```python
from build123d import *

# Parameters (mm, degrees)
EXTRUDE_DEPTH    = 5
EXTRUDE001_DEPTH = 25
EXTRUDE002_DEPTH = 22


with BuildPart() as extrude_body:
    # Sketch → Extrude (new body)
    with BuildSketch(Plane.XY):
        Polygon((115, 0), (57.5, 99.592921), (-57.5, 99.592921), (-115, 0), (-57.5, -99.592921), (57.5, -99.592921), align=None)
    extrude(amount=EXTRUDE_DEPTH)


with BuildPart() as extrude001:
    # Sketch001 (on Sketch) → Extrude001 (new body)
    with BuildSketch(Plane.XY):
        Polygon((115, 0), (57.5, 99.592921), (-57.5, 99.592921), (-115, 0), (-57.5, -99.592921), (57.5, -99.592921), align=None)
        Polygon((112.5, 0), (56.25, 97.427858), (-56.25, 97.427858), (-112.5, 0), (-56.25, -97.427858), (56.25, -97.427858), align=None, mode=Mode.SUBTRACT)
    extrude(amount=EXTRUDE001_DEPTH)


with BuildPart() as fusion:
    # Sketch002 (on Sketch) → Extrude002 (new body)
    with BuildSketch(Plane.XY):
        Polygon((112.5, 0), (56.25, 97.427858), (-56.25, 97.427858), (-112.5, 0), (-56.25, -97.427858), (56.25, -97.427858), align=None)
        Polygon((111, 0), (55.5, 96.12882), (-55.5, 96.12882), (-111, 0), (-55.5, -96.12882), (55.5, -96.12882), align=None, mode=Mode.SUBTRACT)
    extrude(amount=EXTRUDE002_DEPTH)

    # Fusion: union Extrude body, Extrude001
    add(extrude_body.part)
    add(extrude001.part)


solid = fusion.part
```
Source: CAD feature listing. Evaluate the final solid. Frame: model axes, mm. A direction names the side the tool comes from. Coordinates: 2 decimals unless noted, no trailing zeros. Loops run counter-clockwise (first coordinate to the right, second up) from the corner with the lowest first, then second, coordinate; pieces in that order, holes last. Notation, with made-up numbers: (56, 19.25) -> (79, 19.25) arc R18 cw to (79, 51.25) -> close; hole circle Ø10 at (4, 13.25). An arc over 180 degrees is marked (long way). One line per item, written item: value. Start each with the question number.
Q1. Section query B-B, the plane x = 18. Return the cut outline in (y, z), and give its area (3 significant figures).
Q2. Line query: line 1 along Y through (x, z) = (-45, 5.25); line 2 along Y through (x, z) = (56, 22.5); line 3 along Z through (x, y) = (18, 14). Output: solid intervals per line, ascending.
Q3. Mould query, pull axis Y, two halves, no side actions, for faces 1 (the face through (-83.64, -47.39, 13.38)), 2 (the face through (86.65, 49.1, 12.32)), 3 (the face through (-2, 1, 0)). Classes: pulls with the +Y half, pulls with the -Y half, needs draft (parallel to the pull), parting line crosses it, or undercut.
Q4. Contact query for flat-ended pins moving along their axis: P1, Ø8, axis at x = 67, z = 17.5, coming from the +Y side; P2, Ø8, axis at y = -11.5, z = 2.5, coming from the +X side; P3, Ø5, axis at x = 89, z = 22.5, coming from the +Y side. Output: stop coordinate, or through.
Q5. Section query C-C, the plane y = -69. Return the cut outline in (x, z).
Q6. Set-up query: faces 4 (the face through (84.77, 48.03, 23.48)), 5 (the face through (-85.85, 50.49, 12.32)). Return all of +Z, -Z, +X, -X, +Y, -Y with unobstructed straight access to the full face (end or side cutting, diameter ignored); none if empty.
Q7. Section query A-A, the plane z = 19.25. Return the cut outline in (x, y), and give its area (3 significant figures).
Results:
1. outline: (-99.59, 0) -> (99.59, 0) -> (99.59, 25) -> (97.43, 25) -> (97.43, 22) -> (96.13, 22) -> (96.13, 5) -> (-96.13, 5) -> (-96.13, 22) -> (-97.43, 22) -> (-97.43, 25) -> (-99.59, 25) -> close
1. area: 1,130 mm^2
2. line 1: -99.59 to -96.13, 96.13 to 99.59
2. line 2: -99.59 to -97.43, 97.43 to 99.59
2. line 3: 0 to 5
3. face 1: undercut
3. face 2: pulls with the +Y half
3. face 3: needs draft
4. P1: y = 90.07
4. P2: x = 110.67
4. P3: y = 49.36
5. outline: (-75.16, 0) -> (75.16, 0) -> (75.16, 25) -> (72.66, 25) -> (72.66, 22) -> (71.16, 22) -> (71.16, 5) -> (-71.16, 5) -> (-71.16, 22) -> (-72.66, 22) -> (-72.66, 25) -> (-75.16, 25) -> close
6. face 4: +Z
6. face 5: +Z, -Z, -X, +Y
7. outline: (-115, 0) -> (-57.5, -99.59) -> (57.5, -99.59) -> (115, 0) -> (57.5, 99.59) -> (-57.5, 99.59) -> close; hole (-111, 0) -> (-55.5, -96.13) -> (55.5, -96.13) -> (111, 0) -> (55.5, 96.13) -> (-55.5, 96.13) -> close
7. area: 2,350 mm^2
